Check sheet for the modelled part. Datum: model origin and axes. Units: mm. Round coordinates to 2 decimals unless told otherwise and drop trailing zeros. Write each loop counter-clockwise with the first axis right and the second up, starting at its lowest first coordinate (ties: lowest second). Pieces come first, ordered by that corner, then holes. Notation, with made-up numbers: M -5,71 L 40,71 A35 cw 40,109 Z; hole C -3.75,24.25 d3. An arc over 180 degrees is marked long. One line per item, written item: value.
Autodesk Inventor part; units mm, degrees
ref_plane "Start Plane" through (0, 0, 0) normal (1, 0, 0) x (0, 1, 0)
ref_plane "XZ Plane" through (0, 0, 0) normal (0, 1, 0) x (-1, 0, 0)
ref_plane "XY Plane" through (0, 0, 0) normal (0, 0, 1) x (1, 0, 0)
sketch "Main Sketch" plane through (0, 0, 0) normal (0, 0, 1) x (1, 0, 0)
  line L0 (0, 0) -> (26.101, 0)
  line L1 (0, 0) -> (0, 0.375)
  line L2 (0.25, 0.375) -> (0.25, 0.25)
  line L3 (0, 0.375) -> (0.25, 0.375)
  line L4 (5.715, 0.25) -> (5.715, 0.5)
  line L5 (0.25, 0.25) -> (5.715, 0.25)
  line L6 (7.932, 0.5) -> (7.932, 0.25)
  line L7 (5.715, 0.5) -> (7.932, 0.5)
  line L8 (7.932, 0.25) -> (12.804, 0.25)
  line L9 (13.351, 0.5) -> (13.351, 0.25)
  line L10 (12.804, 0.5) -> (13.351, 0.5)
  line L11 (13.351, 0.25) -> (25.851, 0.25)
  line L12 (25.851, 0.25) -> (25.851, 0.375)
  line L13 (26.101, 0.375) -> (26.101, 0)
  line L14 (25.851, 0.375) -> (26.101, 0.375)
  line L15 (12.804, 0.25) -> (12.804, 0.5)
  dimension "d3" = 0.75
  dimension "d6" = 0.5
  dimension "d7" = 1
  dimension "d8" = 0.5
  dimension "d9" = 1
  dimension "d10" = 0.5
  dimension "d11" = 0.75
revolve "Revolution1" add sketch "Main Sketch" angle 360 about axis through (0, 0, 0) along (1, 0, 0)
fillet "Fillet1" [suppressed]
equation "\"Length\" = 26.101"
properties part number "Shaft" material "Steel"
Q1. Sectioned sample at A-A on z = 0. Enter the section's corners in (x, y) (3 decimals), and give its area (3 significant figures).
Completed:
outline: M 0,-0.375 L 0.25,-0.375 L 0.25,-0.25 L 5.715,-0.25 L 5.715,-0.5 L 7.932,-0.5 L 7.932,-0.25 L 12.804,-0.25 L 12.804,-0.5 L 13.351,-0.5 L 13.351,-0.25 L 25.851,-0.25 L 25.851,-0.375 L 26.101,-0.375 L 26.101,0.375 L 25.851,0.375 L 25.851,0.25 L 13.351,0.25 L 13.351,0.5 L 12.804,0.5 L 12.804,0.25 L 7.932,0.25 L 7.932,0.5 L 5.715,0.5 L 5.715,0.25 L 0.25,0.25 L 0.25,0.375 L 0,0.375 Z
area: 14.6 mm^2
Q2. Scan lines: line 1 (X direction, y = -0.25, z = 0.2) (3 decimals); line 2 (X direction, y = 0.4, z = 0.15) (3 decimals); line 3 (Y direction, x = 12.25, z = 0.05). Record each from-to range of solid material in increasing order. Write a range as [from, to].
Completed:
line 1: [0, 0.25], [5.715, 7.932], [12.804, 13.351], [25.851, 26.101]
line 2: [5.715, 7.932], [12.804, 13.351]
line 3: [-0.24, 0.24]
Q3. Sectioned sample at C-C on x = 4. Enter the section's corners in (y, z).
Completed:
outline: C 0,0 d0.5
